```python
from build123d import *

# Parameters (mm, degrees)
F0_W      = 36
F0_H      = 24
F1_DEPTH  = 21.5
F3_DEPTH  = 4
F4_R      = 1.5
F5_DEPTH  = 6
F6_W      = 2
F6_H      = 22
F6_R      = 1.75
F7_DEPTH  = 26.001
F8_R      = 3.5
F9_DEPTH  = 15
F10_R     = 1.5
F11_DEPTH = 6
F12_R     = 1.5
F13_DEPTH = 6
F15_DEPTH = 24.001
F16_W     = 2
F16_H     = 5
F17_DEPTH = 25
F18_W     = 34
F18_H     = 5
F19_DEPTH = 25
F20_W     = 80
F20_H     = 20
F21_DEPTH = 5
F22_W     = 15
F22_H     = 5
F23_DEPTH = 30
F24_W     = 80
F24_H     = 10
F25_DEPTH = 5.001


with BuildPart() as f1:
    # F0 (on Front) → F1 (new body)
    with BuildSketch(Plane.XZ):
        Rectangle(F0_W, F0_H)
    extrude(amount=F1_DEPTH)

    # F2 (on face) → F3 (join)
    with BuildSketch(Plane(origin=(-18, 0, 0), x_dir=(0, -1, 0), z_dir=(-1, 0, 0))):
        Polygon((0, -4), (0, 4), (-4.5, 4), (-4.5, 1.127949), (-3.5, 0.86), (-2.3, 0.86), (-2.3, -0.86), (-3.5, -0.86), (-4.5, -1.127949), (-4.5, -4), align=None)
    extrude(amount=-F3_DEPTH)

    # F4 (on face) → F5 (cut)
    with BuildSketch(Plane.XZ.offset(21.5)):
        with Locations((-12, 0)):
            Circle(F4_R)
        with Locations((2, 0)):
            Circle(F4_R)
    extrude(amount=-F5_DEPTH, mode=Mode.SUBTRACT)

    # F6 (on face) → F7 (cut, through all)
    with BuildSketch(Plane.XZ.offset(21.5)):
        with Locations((17, 1)):
            Rectangle(F6_W, F6_H)
        with Locations((-5, 0)):
            Circle(F6_R)
    extrude(amount=-F7_DEPTH, mode=Mode.SUBTRACT)

    # F8 (on face) → F9 (cut)
    with BuildSketch(Plane.XZ.offset(21.5)):
        with Locations((-5, 0)):
            Circle(F8_R)
    extrude(amount=-F9_DEPTH, mode=Mode.SUBTRACT)

    # F10 (on face) → F11 (cut)
    with BuildSketch(Plane(origin=(0, 0, -12), x_dir=(1, 0, 0), z_dir=(0, 0, -1))):
        with Locations((12, 9.5)):
            Circle(F10_R)
    extrude(amount=-F11_DEPTH, mode=Mode.SUBTRACT)

    # F12 (on face) → F13 (cut)
    with BuildSketch(Plane(origin=(0, 0, 0), x_dir=(-1, 0, 0), z_dir=(0, 1, 0))):
        with Locations((-12, 0)):
            Circle(F12_R)
    extrude(amount=-F13_DEPTH, mode=Mode.SUBTRACT)

    # F14 (on face) → F15 (cut, through all)
    with BuildSketch(Plane.XY.offset(12)):
        Polygon((-18, 4.5), (-18, -16.5), (18, -16.5), (18, 0), (16, 0), (-14, 0), (-14, 4.5), align=None)
    extrude(amount=-F15_DEPTH, mode=Mode.SUBTRACT)

    # F16 (on face) → F17 (cut)
    with BuildSketch(Plane.XY.offset(-10)):
        with Locations((17, -19)):
            Rectangle(F16_W, F16_H)
    extrude(amount=-F17_DEPTH, mode=Mode.SUBTRACT)

    # F18 (on face) → F19 (join)
    with BuildSketch(Plane.XY.offset(12)):
        with Locations((-1, -19)):
            Rectangle(F18_W, F18_H)
    extrude(amount=F19_DEPTH)

    # F20 (on face) → F21 (join)
    with BuildSketch(Plane.XZ.offset(21.5)):
        with Locations((22, 27)):
            Rectangle(F20_W, F20_H)
    extrude(amount=-F21_DEPTH)

    # F22 (on face) → F23 (join)
    with BuildSketch(Plane(origin=(0, 0, 17), x_dir=(1, 0, 0), z_dir=(0, 0, -1))):
        with Locations((54.5, 19)):
            Rectangle(F22_W, F22_H)
    extrude(amount=F23_DEPTH)

    # F24 (on face) → F25 (cut, through all)
    with BuildSketch(Plane.XZ.offset(21.5)):
        with Locations((22, 32)):
            Rectangle(F24_W, F24_H)
    extrude(amount=-F25_DEPTH, mode=Mode.SUBTRACT)


solid = f1.part
```
Part model, mm, in its own coordinate system. A direction names the side the tool comes from. Give positions to 0.01 mm unless a question says otherwise; leave off trailing zeros. Write each loop counter-clockwise with the first axis right and the second up, starting at its lowest first coordinate (ties: lowest second). Pieces come first, ordered by that corner, then holes. Notation, with made-up numbers: (-32, -34) -> (-19, -34) arc R19 cw to (-19, -4) -> close; hole circle Ø7 at (55.25, 30.25). An arc over 180 degrees is marked (long way). Put each result on its own line as item: value. Start each with the question number.
Item 1: Cut at B-B (z = 5.5). List the corners of the cut face in (x, y).
Item 2: Cut at D-D (y = -20.05). List the corners of the cut face in (x, z).
Item 3: Which spindle directions (+Z, -Z, +X, -X, +Y, -Y) get a long thin tool onto all of the face, cutting with end or side? Do faces 1 (the face through (31, -19, 17)), 2 (the face through (-13.5, -19.04, 0.07)). Say none if no direction does.
Item 4: Wall check: L1, parallel to Z at x = -12, y = -18.5; L2, parallel to Z at x = -5, y = -18.9; L3, parallel to X at y = -19.7, z = 7. Give the ranges that are in metal, low to high. Write a range as [from, to].
Item 5: Cut at C-C (z = 0). List the corners of the cut face in (x, y), then the cut area to 3 significant figures.
Item 6: Pin check, flat tips, straight feed: pin 1 Ø1.5 at (x, y) = (39, -19) entering from -Z; pin 2 Ø1.5 at (x, y) = (6.5, -19) entering from -Z. Stop position of each tip, or through.
Item 7: Cut at A-A (x = -5). List the corners of the cut face in (y, z), then the cut area to 3 significant figures.
Item 8: Pull direction X, two halves, no side cores. Call faces 3 (the face through (62, -19, 7)), 4 (the face through (-1.767, -19.035, -1.341)), 5 (the face through (-1, -19, -12)): pulls with the +X half, pulls with the -X half, needs draft (parallel to the pull), parting line crosses it, or undercut.
Answer list:
1. outline: (-18, -21.5) -> (16, -21.5) -> (16, -16.5) -> (-18, -16.5) -> close; (47, -21.5) -> (62, -21.5) -> (62, -16.5) -> (47, -16.5) -> close
2. outline: (-18, -12) -> (16, -12) -> (16, 17) -> (47, 17) -> (47, -13) -> (62, -13) -> (62, 27) -> (-18, 27) -> close; hole circle Ø3 at (-12, 0); hole circle Ø7 at (-5, 0); hole circle Ø3 at (2, 0)
3. face 1: -Z, +Y, -Y
3. face 2: +Y, -Y
4. L1: z = [-12, -1.5], [1.5, 27]
4. L2: z = [-12, -3.5], [3.5, 27]
4. L3: x = [-18, 16], [47, 62]
5. outline: (-18, -21.5) -> (-13.5, -21.5) -> (-13.5, -16.5) -> (-18, -16.5) -> close; (-10.5, -21.5) -> (-8.5, -21.5) -> (-8.5, -16.5) -> (-10.5, -16.5) -> close; (-1.5, -21.5) -> (0.5, -21.5) -> (0.5, -16.5) -> (-1.5, -16.5) -> close; (3.5, -21.5) -> (16, -21.5) -> (16, -16.5) -> (3.5, -16.5) -> close; (47, -21.5) -> (62, -21.5) -> (62, -16.5) -> (47, -16.5) -> close
5. area: 180 mm2
6. pin 1: stops at z = 17
6. pin 2: stops at z = -12
7. outline: (-21.5, -12) -> (-16.5, -12) -> (-16.5, -3.5) -> (-21.5, -3.5) -> close; (-21.5, 3.5) -> (-16.5, 3.5) -> (-16.5, 27) -> (-21.5, 27) -> close
7. area: 160 mm2
8. face 3: pulls with the +X half
8. face 4: undercut
8. face 5: needs draft
